Geometry: final body of the model. Coordinates: model frame, mm. A direction names the side the tool comes from. Round coordinates to 2 decimals unless told otherwise and drop trailing zeros. Write each loop counter-clockwise with the first axis right and the second up, starting at its lowest first coordinate (ties: lowest second). Pieces come first, ordered by that corner, then holes. Notation, with made-up numbers: (48, 21) - (92, 21) arc R9 cw to (92, 28) - close; hole circle Ø2 at (43.25, -30). An arc over 180 degrees is marked (long way). Use a Markdown table: item, result. Add a question column.
```python
from build123d import *

# Parameters (mm, degrees)
SKETCH1_W           = 25.4
SKETCH1_H           = 10.16
BOSS_EXTRUDE2_DEPTH = 0.254
SKETCH2_R           = 2.54
BOSS_EXTRUDE3_DEPTH = 2.54
SKETCH3_W           = 2.54
SKETCH3_H           = 10.16
BOSS_EXTRUDE4_DEPTH = 10.16
SKETCH4_R           = 0.762
CUT_EXTRUDE2_DEPTH  = 25.4


with BuildPart() as part:
    # Sketch1 → Boss-Extrude2 (new body)
    with BuildSketch(Plane(origin=(0, 0, 0), x_dir=(1, 0, 0), z_dir=(0, 1, 0))):
        with Locations((12.7, -5.08)):
            Rectangle(SKETCH1_W, SKETCH1_H)
    extrude(amount=BOSS_EXTRUDE2_DEPTH)

    # Sketch2 → Boss-Extrude3 (add)
    with BuildSketch(Plane(origin=(0, 0.254, 0), x_dir=(1, 0, 0), z_dir=(0, 1, 0))):
        with Locations((12.7, -5.08)):
            Circle(SKETCH2_R)
    extrude(amount=BOSS_EXTRUDE3_DEPTH)

    # Sketch3 → Boss-Extrude4 (add)
    with BuildSketch(Plane(origin=(0, 0.254, 0), x_dir=(1, 0, 0), z_dir=(0, 1, 0))):
        with Locations((1.27, -5.08)):
            Rectangle(SKETCH3_W, SKETCH3_H)
        with Locations((24.13, -5.08)):
            Rectangle(SKETCH3_W, SKETCH3_H)
    extrude(amount=-BOSS_EXTRUDE4_DEPTH)

    # Sketch4 → Cut-Extrude2 (cut)
    with BuildSketch(Plane.ZY):
        with Locations((5.08, -7.366)):
            Circle(SKETCH4_R)
    extrude(amount=-CUT_EXTRUDE2_DEPTH, mode=Mode.SUBTRACT)


solid = part.part
```
1) Set-up query: faces 5 (the flat face through (2.54, -5, 5)), 6 (the cylindrical face through (10.83, 1.51, 3.36)), 7 (the flat face through (1, -9.906, 5)). Return all of +Z, -Z, +X, -X, +Y, -Y with unobstructed straight access to the full face (end or side cutting, diameter ignored); none if empty.
2) Draft query along Y for faces 1 (the cylindrical face through (1.25, -8.11, 4.91)), 2 (the flat face through (13, 0, 5)), 3 (the cylindrical face through (24.11, -8.11, 4.91)), 4 (the flat face through (22.86, -5, 5)). Return one class per face: released by +Y, released by -Y, zero draft, split by the parting line, or undercut.
3) Section B-B, the plane x = 12.7. Return the cut outline in (y, z), then the cut area to 3 significant figures.
4) Section D-D, the plane z = 9. Return the cut outline in (x, y).
5) Pin query (flat end, axial travel): P1, Ø2, axis at x = 13, z = 2, coming from the -Y side; P2, Ø5, axis at y = -6.5, z = 7.5, coming from the -X side; P3, Ø5, axis at x = 6, y = -7, coming from the -Z side. Return the tip coordinate at first contact, or that it passes through.
6) Material intervals for L1, parallel to Y at x = 1.45, z = 5.08; L2, parallel to X at y = -4.5, z = 9.25; L3, parallel to Y at x = 1.5, z = 8, sorted ascending. Write a range as from..to.
7) Section C-C, the plane y = -2. Return the cut outline in (x, z), then the cut area to 3 significant figures.
8) Section A-A, the plane z = 5.08. Return the cut outline in (x, y), then the cut area to 3 significant figures.
Output values:
| question | item | result |
|---|---|---|
| 1 | face 5 | +Z, -Z, -Y |
| 1 | face 6 | +Y |
| 1 | face 7 | +Z, -Z, +X, -X, -Y |
| 2 | face 1 | undercut |
| 2 | face 2 | released by -Y |
| 2 | face 3 | undercut |
| 2 | face 4 | zero draft |
| 3 | outline | (0, 0) - (0.25, 0) - (0.25, 2.54) - (2.79, 2.54) - (2.79, 7.62) - (0.25, 7.62) - (0.25, 10.16) - (0, 10.16) - close |
| 3 | area | 15.5 mm^2 |
| 4 | outline | (0, -9.91) - (2.54, -9.91) - (2.54, 0) - (22.86, 0) - (22.86, -9.91) - (25.4, -9.91) - (25.4, 0.25) - (0, 0.25) - close |
| 5 | P1 | stops at y = 0 |
| 5 | P2 | stops at x = 0 |
| 5 | P3 | passes through |
| 6 | L1 | y = -9.91..-8.13, -6.6..0.25 |
| 6 | L2 | x = 0..2.54, 22.86..25.4 |
| 6 | L3 | y = -9.91..0.25 |
| 7 | outline | (0, 0) - (2.54, 0) - (2.54, 10.16) - (0, 10.16) - close; (22.86, 0) - (25.4, 0) - (25.4, 10.16) - (22.86, 10.16) - close |
| 7 | area | 51.6 mm^2 |
| 8 | outline | (0, -9.91) - (2.54, -9.91) - (2.54, -8.13) - (0, -8.13) - close; (0, -6.6) - (2.54, -6.6) - (2.54, 0) - (22.86, 0) - (22.86, -6.6) - (25.4, -6.6) - (25.4, 0.25) - (15.24, 0.25) - (15.24, 2.79) - (10.16, 2.79) - (10.16, 0.25) - (0, 0.25) - close; (22.86, -9.91) - (25.4, -9.91) - (25.4, -8.13) - (22.86, -8.13) - close |
| 8 | area | 61.9 mm^2 |
